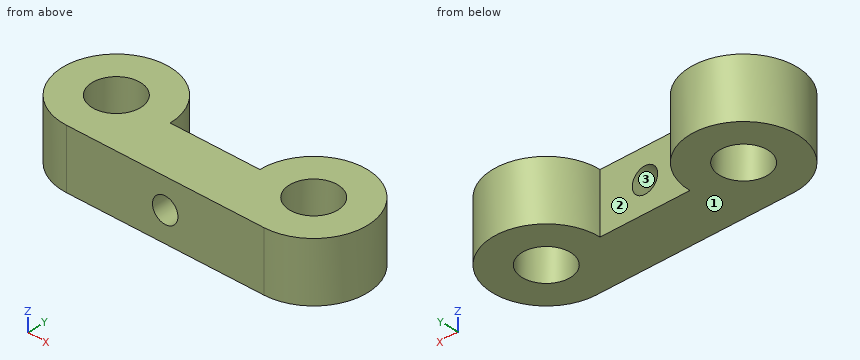
```python
from build123d import *

# Parameters (mm, degrees)
ESBO_O1_R                = 4.05
RESSALTO_EXTRUS_O1_DEPTH = 10
ESBO_O2_R                = 2.125
CORTE_EXTRUS_O1_DEPTH    = 10


with BuildPart() as part:
    # Esboço1 → Ressalto-extrusão1 (new body)
    with BuildSketch(Plane.XY):
        with BuildLine():
            Line((-16.5, -9), (16.5, -9))
            ThreePointArc((16.5, -9), (22.863961031, 6.363961031), (7.5, 0))
            Line((7.5, 0), (-7.5, 0))
            ThreePointArc((-7.5, 0), (-22.863961031, 6.363961031), (-16.5, -9))
        make_face()
        with Locations((-16.5, 0)):
            Circle(ESBO_O1_R, mode=Mode.SUBTRACT)
        with Locations((16.5, 0)):
            Circle(ESBO_O1_R, mode=Mode.SUBTRACT)
    extrude(amount=RESSALTO_EXTRUS_O1_DEPTH)

    # Esboço2 → Corte-extrusão1 (cut)
    with BuildSketch(Plane(origin=(0, 0, 0), x_dir=(1, 0, 0), z_dir=(0, 1, 0))):
        with Locations((0, -5)):
            Circle(ESBO_O2_R)
    extrude(amount=-CORTE_EXTRUS_O1_DEPTH, mode=Mode.SUBTRACT)


solid = part.part
```
Can you work these out from the model? Positions are in its coordinate system, mm. Face numbers are marked on the shaded views. Coordinates: 2 decimals unless noted, no trailing zeros. Loops run counter-clockwise (first coordinate to the right, second up) from the corner with the lowest first, then second, coordinate; pieces in that order, holes last.
1) For pin 1 (1 mm diameter, centred on x = -14, z = 2.5, fed in from +Y), with a flat end and sliding along its axis, tell me the tip position at first contact or that it passes through.
2) Thinking about a two-plate mould opening in Z: for the marked faces 1, 2 and 3, which applies, pulls with the +Z half, pulls with the -Z half, needs draft (parallel to the pull), parting line crosses it, or undercut?
3) Imagine slicing it at D-D on y = 2.5. List the corners of the cut face in (x, z) for me, plus the area to 3 significant figures.
4) Imagine slicing it at B-B on x = 0. List the corners of the cut face in (y, z) for me (3 decimals).
5) I need wall thicknesses on probe 1 along Z at (x, y) = (0, -6.5) (3 decimals); probe 2 along X at (y, z) = (3, 3.25); probe 3 along X at (y, z) = (-1.25, 9). Which ranges of each line are inside material? Lowest first, please.
6) Imagine slicing it at A-A on z = 5. List the corners of the cut face in (x, y) for me (3 decimals).
7) Imagine slicing it at C-C on y = -2.75. List the corners of the cut face in (x, z) for me (3 decimals), plus the area to 3 significant figures.
Completed:
1. pin 1: stops at y = 8.77
2. face 1: pulls with the -Z half
2. face 2: needs draft
2. face 3: undercut
3. outline: (-25.15, 0) - (-19.69, 0) - (-19.69, 10) - (-25.15, 10) - close; (-13.31, 0) - (-7.85, 0) - (-7.85, 10) - (-13.31, 10) - close; (7.85, 0) - (13.31, 0) - (13.31, 10) - (7.85, 10) - close; (19.69, 0) - (25.15, 0) - (25.15, 10) - (19.69, 10) - close
3. area: 218 mm2
4. outline: (-9, 0) - (0, 0) - (0, 2.875) - (-9, 2.875) - close; (-9, 7.125) - (0, 7.125) - (0, 10) - (-9, 10) - close
5. probe 1: z = 0 to 2.875, 7.125 to 10
5. probe 2: x = -24.99 to -19.22, -13.78 to -8.01, 8.01 to 13.78, 19.22 to 24.99
5. probe 3: x = -25.41 to -20.35, -12.65 to 12.65, 20.35 to 25.41
6. outline: (-16.5, -9) - (-2.125, -9) - (-2.125, 0) - (-7.5, 0) arc R9 ccw (long way) to start; (2.125, -9) - (16.5, -9) arc R9 ccw (long way) to (7.5, 0) - (2.125, 0) - close; hole circle Ø8.1 at (-16.5, 0); hole circle Ø8.1 at (16.5, 0)
7. outline: (-25.07, 0) - (-19.473, 0) - (-19.473, 10) - (-25.07, 10) - close; (-13.527, 0) - (13.527, 0) - (13.527, 10) - (-13.527, 10) - close; (19.473, 0) - (25.07, 0) - (25.07, 10) - (19.473, 10) - close; hole circle Ø4.25 at (0, 5)
7. area: 368 mm2
